from build123d import *

# Parameters (mm, degrees)
F0_W     = 355.6
F0_H     = 127
F1_DEPTH = 152.4
F2_W     = 266.7
F2_H     = 12.7
F3_DEPTH = 152.4
F4_W     = 12.7
F4_H     = 12.7
F4_H_2   = 6.35
F4_H_3   = 38.1
F5_DEPTH = 152.4
F6_W     = 12.7
F6_H     = 12.7
F6_W_2   = 6.35
F6_W_3   = 38.1
F7_DEPTH = 342.9


with BuildPart() as f1:
    # F0 (on Top) → F1 (new body)
    with BuildSketch(Plane.XY):
        Rectangle(F0_W, F0_H)
    extrude(amount=-F1_DEPTH)

    # F2 (on face) → F3 (cut)
    with BuildSketch(Plane.XY):
        Polygon((152.4, -63.5), (165.1, -63.5), (171.45, -50.8), (146.05, -50.8), align=None)
        with Locations((6.35, -57.15)):
            Rectangle(F2_W, F2_H)
        Polygon((-139.7, -63.5), (-133.35, -50.8), (-158.75, -50.8), (-152.4, -63.5), align=None)
    extrude(amount=-F3_DEPTH, mode=Mode.SUBTRACT)

    # F4 (on face) → F5 (cut)
    with BuildSketch(Plane.XY):
        with Locations((-171.45, -57.15)):
            Rectangle(F4_W, F4_H)
        Polygon((-165.1, 57.15), (-177.8, 57.15), (-177.8, 50.8), align=None)
        with Locations((-171.45, 60.325)):
            Rectangle(F4_W, F4_H_2)
        Polygon((-177.8, 31.75), (-165.1, 31.75), (-177.8, 38.1), align=None)
        with Locations((-171.45, 28.575)):
            Rectangle(F4_W, F4_H_2)
        with Locations((-171.45, -15.875)):
            Rectangle(F4_W, F4_H_2)
        Polygon((-177.8, -25.4), (-165.1, -19.05), (-177.8, -19.05), align=None)
        Polygon((-177.8, -44.45), (-165.1, -44.45), (-177.8, -38.1), align=None)
        with Locations((-171.45, -47.625)):
            Rectangle(F4_W, F4_H_2)
        with Locations((-171.45, 6.35)):
            Rectangle(F4_W, F4_H_3)
        Polygon((-165.1, -44.45), (-165.1, -19.05), (-177.8, -25.4), (-177.8, -38.1), align=None)
        Polygon((-165.1, 31.75), (-165.1, 57.15), (-177.8, 50.8), (-177.8, 38.1), align=None)
    extrude(amount=-F5_DEPTH, mode=Mode.SUBTRACT)

    # F6 (on face) → F7 (cut)
    with BuildSketch(Plane.YZ.offset(177.8)):
        with Locations((-57.15, -6.35)):
            Rectangle(F6_W, F6_H)
        with Locations((-47.625, -6.35)):
            Rectangle(F6_W_2, F6_H)
        Polygon((-38.1, -12.7), (-44.45, 0), (-44.45, -12.7), align=None)
        Polygon((-19.05, -12.7), (-19.05, 0), (-25.4, -12.7), align=None)
        with Locations((-15.875, -6.35)):
            Rectangle(F6_W_2, F6_H)
        with Locations((6.35, -6.35)):
            Rectangle(F6_W_3, F6_H)
        with Locations((28.575, -6.35)):
            Rectangle(F6_W_2, F6_H)
        Polygon((38.1, -12.7), (31.75, 0), (31.75, -12.7), align=None)
        Polygon((57.15, -12.7), (57.15, 0), (50.8, -12.7), align=None)
        with Locations((60.325, -6.35)):
            Rectangle(F6_W_2, F6_H)
    extrude(amount=-F7_DEPTH, mode=Mode.SUBTRACT)


solid = f1.part
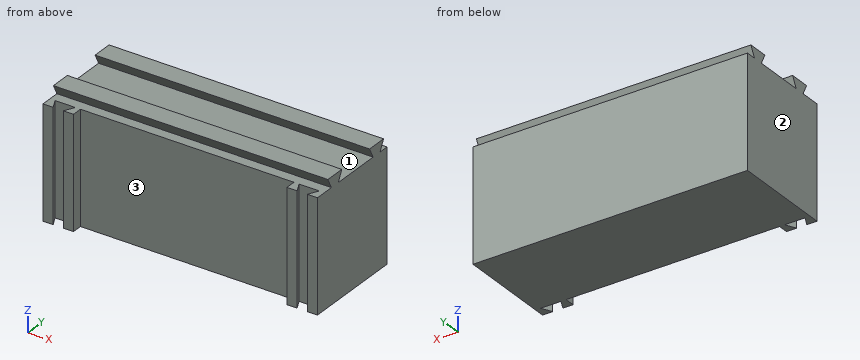
Model file for the job. Use its own axes, mm. Face numbers are marked on the shaded views. A direction names the side the tool comes from. Round coordinates to 2 decimals unless told otherwise and drop trailing zeros. Loops run counter-clockwise (first coordinate to the right, second up) from the corner with the lowest first, then second, coordinate; pieces in that order, holes last.
1. Band-saw the part on A-A, the plane x = 83. List the corners of the cut face in (y, z).
Check values:
outline: (-50.8, -152.4) - (63.5, -152.4) - (63.5, -12.7) - (50.8, -12.7) - (57.15, 0) - (31.75, 0) - (38.1, -12.7) - (-25.4, -12.7) - (-19.05, 0) - (-44.45, 0) - (-38.1, -12.7) - (-50.8, -12.7) - close
2. Band-saw the part on C-C, the plane y = 11.5. List the corners of the cut face in (x, z), and give its area (3 significant figures).
Check values:
outline: (-165.1, -152.4) - (177.8, -152.4) - (177.8, -12.7) - (-165.1, -12.7) - close
area: 47,900 mm2
3. Tool access for the marked faces 1, 2 and 3: list every direction of +Z, -Z, +X, -X, +Y, -Y with a clear straight run to the whole face (end or side of a thin tool).
Check values:
face 1: +X, -X
face 2: +Z, -Z, -X, +Y, -Y
face 3: +Z, -Z, -Y
4. Wall check: probe 1 along Y at (x, z) = (-65, -26); probe 2 along Z at (x, y) = (0.5, -6); probe 3 along Y at (x, z) = (21.5, -7). Give the ranges that are in metal, low to high.
Check values:
probe 1: y = -50.8 to 63.5
probe 2: z = -152.4 to -12.7
probe 3: y = -40.95 to -22.55, 35.25 to 53.65
5. Band-saw the part on B-B, the plane z = -132. List the corners of the cut face in (x, y), and give its area (3 significant figures).
Check values:
outline: (-165.1, -63.5) - (-152.4, -63.5) - (-158.75, -50.8) - (-133.35, -50.8) - (-139.7, -63.5) - (-127, -63.5) - (-127, -50.8) - (139.7, -50.8) - (139.7, -63.5) - (152.4, -63.5) - (146.05, -50.8) - (171.45, -50.8) - (165.1, -63.5) - (177.8, -63.5) - (177.8, 63.5) - (-165.1, 63.5) - close
area: 39,700 mm2
6. Drop flat-ended pins along their axis: P1, Ø7.5, axis at x = -13.5, y = -50.5, coming from the +Z side; P2, Ø12, axis at x = 47.5, z = -128, coming from the -Y side. Give the stop position or say it passes through.
Check values:
P1: stops at z = -12.7
P2: stops at y = -50.8
